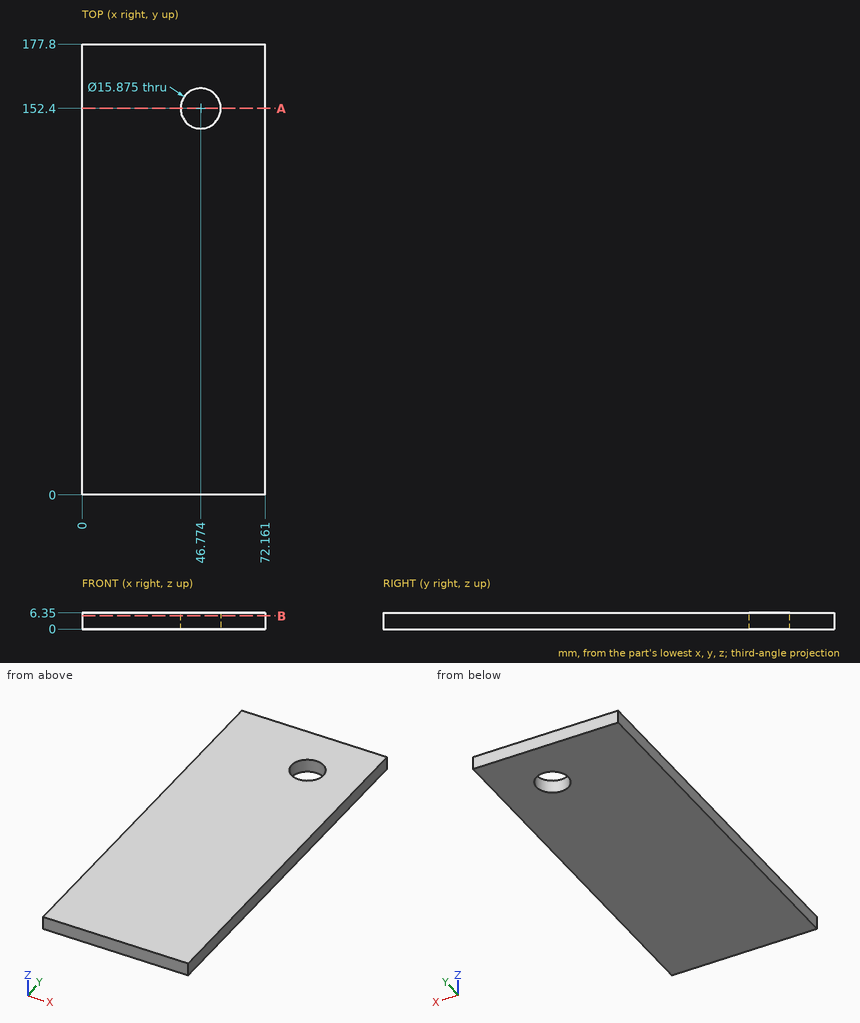
Study the drawing (mm; zero at the part's minimum x, y, z) and answer. Coordinates: 2 decimals unless noted, no trailing zeros. Write each loop counter-clockwise with the first axis right and the second up, starting at its lowest first coordinate (ties: lowest second). Pieces come first, ordered by that corner, then holes. Notation, with made-up numbers: M 37,-24 L 59,-24 A30 cw 59,2 Z; hole C -15.75,16.25 d9. An arc over 180 degrees is marked long. Use one line per item in the form item = value.
Item 1: Find section B-B, the plane z = 5.25. Give the vertices of the cut face in (x, y) (1 decimal), plus the area to 3 significant figures.
Model answer:
outline = M 0,0 L 72.2,0 L 72.2,177.8 L 0,177.8 Z; hole C 46.8,152.4 d15.9
area = 12,600 mm2
Item 2: Find the intervals of material crossed by probe 1 along X at (y, z) = (150, 3.75); probe 2 along Y at (x, z) = (50.5, 4.75), in increasing order.
Model answer:
probe_1 = 0 to 39.21, 54.34 to 72.16
probe_2 = 0 to 145.39, 159.41 to 177.8
Item 3: Find section A-A, the plane y = 152.4. Give the vertices of the cut face in (x, z).
Model answer:
outline = M 0,0 L 38.84,0 L 38.84,6.35 L 0,6.35 Z; M 54.71,0 L 72.16,0 L 72.16,6.35 L 54.71,6.35 Z
